from build123d import *

# Parameters (mm, degrees)
SKETCH1_R           = 4
BOSS_EXTRUDE1_DEPTH = 3.175
FILLET1_R           = 5


with BuildPart() as part:
    # Sketch1 → Boss-Extrude1 (new, symmetric)
    with BuildSketch(Plane(origin=(0, 0, 0), x_dir=(1, 0, 0), z_dir=(0, 1, 0))):
        with BuildLine():
            Line((-78.675, -56.35), (-58.675, -56.35))
            Line((-58.675, -56.35), (-58.675, -50))
            Line((-58.675, -50), (58.675, -50))
            Line((58.675, -50), (58.675, -56.35))
            Line((58.675, -56.35), (78.675, -56.35))
            Line((78.675, -56.35), (78.675, -36.35))
            Line((78.675, -36.35), (72.325, -36.35))
            Line((72.325, -36.35), (72.325, 36.35))
            Line((72.325, 36.35), (78.675, 36.35))
            Line((78.675, 36.35), (78.675, 56.35))
            Line((78.675, 56.35), (62.325, 56.35))
            Line((62.325, 56.35), (62.325, 50))
            Line((62.325, 50), (42.325, 50))
            ThreePointArc((42.325, 50), (12.399475155, -22.753839327), (-64.675, -7))
            Line((-64.675, -7), (-78.675, -7))
            Line((-78.675, -7), (-78.675, -56.35))
        make_face()
        with Locations(Location((-71.675, -41, 0), (0, 0, 270))):
            Circle(SKETCH1_R, mode=Mode.SUBTRACT)
        with Locations(Location((-71.675, -14, 0), (0, 0, 270))):
            Circle(SKETCH1_R, mode=Mode.SUBTRACT)
    extrude(amount=BOSS_EXTRUDE1_DEPTH, both=True)

    # Fillet1
    fillet1_edges = [part.edges().sort_by_distance(p)[0] for p in [
        (-78.675, 0, 7),
        (-64.675, 0, 7),
        (42.325, 0, -50),
    ]]
    fillet(fillet1_edges, radius=FILLET1_R)


solid = part.part
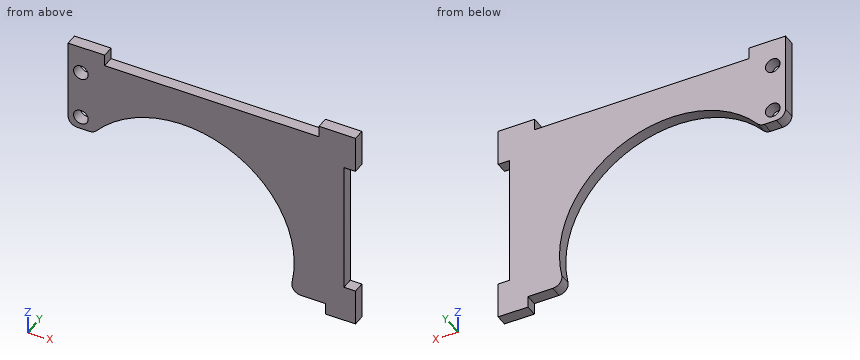
Geometry check sheet. Reference: the model listing, model coordinates, mm. Round coordinates to 2 decimals unless told otherwise and drop trailing zeros. Write each loop counter-clockwise with the first axis right and the second up, starting at its lowest first coordinate (ties: lowest second). Pieces come first, ordered by that corner, then holes. Notation, with made-up numbers: (23.25, 89.25) -> (55.25, 89.25) arc R16 ccw to (55.25, 95.25) -> close; hole circle Ø6 at (44.25, -24.5). An arc over 180 degrees is marked (long way). One line per item, written item: value. Start each with the question number.
(1) Cross-section at B-B, the plane y = 0.25. Record the cut outline in (x, z) (3 decimals), and give its area (3 significant figures).
(2) Cross-section at D-D, the plane x = 15. Record the cut outline in (y, z) (3 decimals).
(3) Cross-section at A-A, the plane z = 41. Record the cut outline in (x, y) (3 decimals).
(4) Cross-section at C-C, the plane z = 14. Record the cut outline in (x, y) (3 decimals).
(5) Go/stop test with flat-tipped pins: pin 1 Ø7 at (x, z) = (-71.675, 41) entering from +Y; pin 2 Ø1.5 at (y, z) = (1.5, 5) entering from +X (3 decimals); pin 3 Ø3 at (y, z) = (-1, -53) entering from -X (3 decimals); pin 4 Ø3 at (x, y) = (-48, 0) entering from -Z. Record where each tip stops, or that it passes through.
(6) Scan lines: line 1 (X direction, y = -1.75, z = 41) (3 decimals); line 2 (Z direction, x = -66.5, y = 1); line 3 (X direction, y = -1, z = 14) (3 decimals). Record each from-to range of solid material in increasing order. Write a range as [from, to].
Answer:
1. outline: (-78.675, 12) arc R5 ccw to (-73.675, 7) -> (-67.011, 7) arc R5 ccw to (-63.234, 8.724) arc R61.712 cw to (43.86, -44.004) arc R5 ccw to (48.76, -50) -> (62.325, -50) -> (62.325, -56.35) -> (78.675, -56.35) -> (78.675, -36.35) -> (72.325, -36.35) -> (72.325, 36.35) -> (78.675, 36.35) -> (78.675, 56.35) -> (58.675, 56.35) -> (58.675, 50) -> (-58.675, 50) -> (-58.675, 56.35) -> (-78.675, 56.35) -> close; hole circle Ø8 at (-71.675, 14); hole circle Ø8 at (-71.675, 41)
1. area: 7,110 mm²
2. outline: (-3.175, 21.287) -> (3.175, 21.287) -> (3.175, 50) -> (-3.175, 50) -> close
3. outline: (-78.675, -3.175) -> (-75.675, -3.175) -> (-75.675, 3.175) -> (-78.675, 3.175) -> close; (-67.675, -3.175) -> (78.675, -3.175) -> (78.675, 3.175) -> (-67.675, 3.175) -> close
4. outline: (-78.675, -3.175) -> (-75.675, -3.175) -> (-75.675, 3.175) -> (-78.675, 3.175) -> close; (-67.675, -3.175) -> (-58.073, -3.175) -> (-58.073, 3.175) -> (-67.675, 3.175) -> close; (24.843, -3.175) -> (72.325, -3.175) -> (72.325, 3.175) -> (24.843, 3.175) -> close
5. pin 1: through
5. pin 2: x = 72.325
5. pin 3: x = 62.325
5. pin 4: z = 20.51
6. line 1: [-78.675, -75.675], [-67.675, 78.675]
6. line 2: [7.03, 56.35]
6. line 3: [-78.675, -75.675], [-67.675, -58.073], [24.843, 72.325]
